The listing builds one solid part. Answer for the finished solid, in the listing's coordinates (mm). A direction names the side the tool comes from. Coordinates: 2 decimals unless noted, no trailing zeros. Order: outer loops, then holes, each group sorted by start corner. A loop starts at its lowest first (then second) coordinate and runs counter-clockwise, first axis right, second up.
from build123d import *

# Parameters (mm, degrees)
F0_W     = 787.4
F0_H     = 584.2
F1_DEPTH = 1447.8
F2_W     = 711.2
F2_H     = 304.8
F3_DEPTH = 546.1
F5_DEPTH = 1016


with BuildPart() as f1:
    # F0 (on Top) → F1 (new body)
    with BuildSketch(Plane.XY):
        with Locations((322.746758, 217.150773)):
            Rectangle(F0_W, F0_H)
    extrude(amount=F1_DEPTH)

    # F2 (on face) → F3 (cut)
    with BuildSketch(Plane.XZ.offset(74.949227)):
        with Locations((322.746758, 1295.4)):
            Rectangle(F2_W, F2_H)
    extrude(amount=-F3_DEPTH, mode=Mode.SUBTRACT)

    # F4 (on face) → F5 (cut)
    with BuildSketch(Plane.XY.offset(1143)):
        with BuildLine():
            ThreePointArc((27.243803, 1.250773), (27.243803, -24.149227), (49.240848, -36.849227))
            Line((49.240848, -36.849227), (164.452667, -36.849227))
            ThreePointArc((164.452667, -36.849227), (186.449712, -24.149227), (186.449712, 1.250773))
            Line((186.449712, 1.250773), (128.843803, 101.027135))
            ThreePointArc((128.843803, 101.027135), (106.846758, 113.727135), (84.849712, 101.027135))
            Line((84.849712, 101.027135), (27.243803, 1.250773))
        make_face()
        with BuildLine():
            ThreePointArc((380.352667, -36.849227), (402.349712, -24.149227), (402.349712, 1.250773))
            Line((402.349712, 1.250773), (344.743803, 101.027135))
            ThreePointArc((344.743803, 101.027135), (322.746758, 113.727135), (300.749712, 101.027135))
            Line((300.749712, 101.027135), (243.143803, 1.250773))
            ThreePointArc((243.143803, 1.250773), (243.143803, -24.149227), (265.140848, -36.849227))
            Line((265.140848, -36.849227), (380.352667, -36.849227))
        make_face()
        with BuildLine():
            ThreePointArc((596.252667, -36.849227), (618.249712, -24.149227), (618.249712, 1.250773))
            Line((618.249712, 1.250773), (560.643803, 101.027135))
            ThreePointArc((560.643803, 101.027135), (538.646758, 113.727135), (516.649712, 101.027135))
            Line((516.649712, 101.027135), (459.043803, 1.250773))
            ThreePointArc((459.043803, 1.250773), (459.043803, -24.149227), (481.040848, -36.849227))
            Line((481.040848, -36.849227), (596.252667, -36.849227))
        make_face()
        with BuildLine():
            Line((272.760662, 179.894812), (157.548843, 179.894812))
            ThreePointArc((157.548843, 179.894812), (135.551798, 167.194812), (135.551798, 141.794812))
            Line((135.551798, 141.794812), (193.157707, 42.01845))
            ThreePointArc((193.157707, 42.01845), (215.154753, 29.31845), (237.151798, 42.01845))
            Line((237.151798, 42.01845), (294.757707, 141.794812))
            ThreePointArc((294.757707, 141.794812), (294.757707, 167.194812), (272.760662, 179.894812))
        make_face()
        with BuildLine():
            ThreePointArc((509.941717, 141.794812), (509.941717, 167.194812), (487.944672, 179.894812))
            Line((487.944672, 179.894812), (372.732853, 179.894812))
            ThreePointArc((372.732853, 179.894812), (350.735808, 167.194812), (350.735808, 141.794812))
            Line((350.735808, 141.794812), (408.341717, 42.01845))
            ThreePointArc((408.341717, 42.01845), (430.338762, 29.31845), (452.335808, 42.01845))
            Line((452.335808, 42.01845), (509.941717, 141.794812))
        make_face()
        with BuildLine():
            Line((164.452667, 433.050773), (49.240848, 433.050773))
            ThreePointArc((49.240848, 433.050773), (27.243803, 420.350773), (27.243803, 394.950773))
            Line((27.243803, 394.950773), (84.849712, 295.174411))
            ThreePointArc((84.849712, 295.174411), (106.846758, 282.474411), (128.843803, 295.174411))
            Line((128.843803, 295.174411), (186.449712, 394.950773))
            ThreePointArc((186.449712, 394.950773), (186.449712, 420.350773), (164.452667, 433.050773))
        make_face()
        with BuildLine():
            Line((560.643803, 295.174411), (618.249712, 394.950773))
            ThreePointArc((618.249712, 394.950773), (618.249712, 420.350773), (596.252667, 433.050773))
            Line((596.252667, 433.050773), (481.040848, 433.050773))
            ThreePointArc((481.040848, 433.050773), (459.043803, 420.350773), (459.043803, 394.950773))
            Line((459.043803, 394.950773), (516.649712, 295.174411))
            ThreePointArc((516.649712, 295.174411), (538.646758, 282.474411), (560.643803, 295.174411))
        make_face()
        with BuildLine():
            ThreePointArc((237.151798, 354.183096), (215.154753, 366.883096), (193.157707, 354.183096))
            Line((193.157707, 354.183096), (135.551798, 254.406734))
            ThreePointArc((135.551798, 254.406734), (135.551798, 229.006734), (157.548843, 216.306734))
            Line((157.548843, 216.306734), (272.760662, 216.306734))
            ThreePointArc((272.760662, 216.306734), (294.757707, 229.006734), (294.757707, 254.406734))
            Line((294.757707, 254.406734), (237.151798, 354.183096))
        make_face()
        with BuildLine():
            Line((408.341717, 354.183096), (350.735808, 254.406734))
            ThreePointArc((350.735808, 254.406734), (350.735808, 229.006734), (372.732853, 216.306734))
            Line((372.732853, 216.306734), (487.944672, 216.306734))
            ThreePointArc((487.944672, 216.306734), (509.941717, 229.006734), (509.941717, 254.406734))
            Line((509.941717, 254.406734), (452.335808, 354.183096))
            ThreePointArc((452.335808, 354.183096), (430.338762, 366.883096), (408.341717, 354.183096))
        make_face()
        with BuildLine():
            ThreePointArc((265.140848, 433.050773), (243.143803, 420.350773), (243.143803, 394.950773))
            Line((243.143803, 394.950773), (300.749712, 295.174411))
            ThreePointArc((300.749712, 295.174411), (322.746758, 282.474411), (344.743803, 295.174411))
            Line((344.743803, 295.174411), (402.349712, 394.950773))
            ThreePointArc((402.349712, 394.950773), (402.349712, 420.350773), (380.352667, 433.050773))
            Line((380.352667, 433.050773), (265.140848, 433.050773))
        make_face()
    extrude(amount=-F5_DEPTH, mode=Mode.SUBTRACT)


solid = f1.part
(1) Find section A-A on x = -13. Determine the outline of the cut face in (y, z).
(2) A tool of negligible diameter and unlimited length cuts with its end or side. For faces 1 (the cylindrical face through (186.63, 420.03, 642.11)), 2 (the flat face through (318, 194, 1143)), 3 (the flat face through (716.447, 213, 714)), from which of +Z, -Z, +X, -X, +Y, -Y can it reach the whole face along a straight path? Write none if from no direction.
(3) Find the intervals of material crossed by probe 1 along X at (y, z) = (407, 969.5); probe 2 along Y at (x, z) = (319, 769); probe 3 along X at (y, z) = (324.5, 1155.5), in increasing order.
(4) Find section D-D on y = 340. Determine the outline of the cut face in (x, z).
(5) The mould has two halves that part along Y. Classify faces 4 (the flat face through (317, -74.949, 553)), 5 (the flat face through (56.45, 51.84, 642.11)), 6 (the flat face through (292, 478, 1447.8)), 7 (the cylindrical face through (186.26, -24.47, 642.11)): pulls with the +Y half, pulls with the -Y half, needs draft (parallel to the pull), parting line crosses it, or undercut.
(6) Given pin 1 Ø12 at (x, y) = (213.5, 233) entering from -Z; pin 2 Ø1 at (x, z) = (148.5, 1263) entering from -Y; pin 3 Ø1 at (x, y) = (92, 198.5) entering from +Z, each flat-ended and moving along its own axis, determine where each tip first touches the part or whether it passes through.
(7) Find section B-B on z = 1308.5. Determine the outline of the cut face in (x, y).
(8) Find section C-C on z = 825.5. Count the separate pieces of the cut face and the enclosed holes in it, then the cut area to 3 significant figures.
Resolved:
1. outline: (-74.95, 0) - (509.25, 0) - (509.25, 1447.8) - (471.15, 1447.8) - (471.15, 1143) - (-74.95, 1143) - close
2. face 1: +Z
2. face 2: +Z, -Y
2. face 3: +Z, -Z, +X, +Y, -Y
3. probe 1: x = -70.95 to 23.85, 189.84 to 239.75, 405.74 to 455.65, 621.64 to 716.45
3. probe 2: y = -74.95 to -36.85, 113.45 to 282.75, 433.05 to 509.25
3. probe 3: x = -70.95 to -32.85, 678.35 to 716.45
4. outline: (-70.95, 0) - (716.45, 0) - (716.45, 1447.8) - (678.35, 1447.8) - (678.35, 1143) - (586.52, 1143) - (586.52, 127) - (490.77, 127) - (490.77, 1143) - (460.52, 1143) - (460.52, 127) - (400.15, 127) - (400.15, 1143) - (370.62, 1143) - (370.62, 127) - (274.87, 127) - (274.87, 1143) - (245.34, 1143) - (245.34, 127) - (184.97, 127) - (184.97, 1143) - (154.72, 1143) - (154.72, 127) - (58.97, 127) - (58.97, 1143) - (-32.85, 1143) - (-32.85, 1447.8) - (-70.95, 1447.8) - close
5. face 4: pulls with the -Y half
5. face 5: undercut
5. face 6: needs draft
5. face 7: undercut
6. pin 1: stops at z = 0
6. pin 2: stops at y = 471.15
6. pin 3: stops at z = 1143
7. outline: (-70.95, -74.95) - (-32.85, -74.95) - (-32.85, 471.15) - (678.35, 471.15) - (678.35, -74.95) - (716.45, -74.95) - (716.45, 509.25) - (-70.95, 509.25) - close
8. separate pieces: 1
8. enclosed holes: 10
8. area: 294,000 mm2
